Work out the finished part from the listing and answer in its coordinate system (mm). A direction names the side the tool comes from. Coordinates: 2 decimals unless noted, no trailing zeros. Write each loop counter-clockwise with the first axis right and the second up, starting at its lowest first coordinate (ties: lowest second). Pieces come first, ordered by that corner, then holes. Notation, with made-up numbers: (-19, 82.5) - (-7, 82.5) arc R26 ccw to (-7, 98.5) - close; hole circle Ø1 at (-3, 60). An arc over 180 degrees is marked (long way). Use a Markdown table: item, result. Add a question column.
(1) Find the intervals of material crossed by line 1 (Y direction, x = -4, z = -0.75); line 2 (X direction, y = 8, z = -1); line 3 (X direction, y = 23, z = -1.75), in increasing order. Write a range as from..to.
(2) The part is cut by section D-D, the plane x = -16. Give the vertices of the cut face in (y, z).
(3) For a pull along X with two mould halves and no side action, classify faces 1 (the face through (-0.75, 35, 2)), 2 (the face through (0, 17, 0)), 3 (the face through (-21, 3, 0)), 4 (the face through (-5, 37.5, 0)) as released by +X, released by -X, zero draft, split by the parting line, or undercut.
(4) The part is cut by section A-A, the plane y = 33. Give the vertices of the cut face in (x, z), then the cut area to 3 significant figures.
(5) The part is cut by section C-C, the plane x = 2. Give the vertices of the cut face in (y, z).
(6) The part is cut by section B-B, the plane z = 0. Give the vertices of the cut face in (x, y), then the cut area to 3 significant figures.
(7) Given pin 1 Ø4.5 at (y, z) = (34.5, 0.5) entering from -X; pin 2 Ø5.5 at (x, z) = (-18, -2.5) entering from +Y; pin 3 Ø4 at (y, z) = (27.5, 3) entering from +X, each flat-ended and moving along its own axis, determine where each tip first touches the part or whether it passes through.
(8) A tool of negligible diameter and unlimited length cuts with its end or side. For faces 5 (the face through (13, 6, 0)), 6 (the face through (0.75, 35, 2)), 7 (the face through (18.747, 3.042, 0.121)), 8 (the face through (-13, 6, 0)), from which of +Z, -Z, +X, -X, +Y, -Y can it reach the whole face along a straight path? Write none if from no direction.
from build123d import *

# Parameters (mm, degrees)
BOSS_EXTRUDE1_DEPTH = 7
SKETCH2_R           = 6
CUT_EXTRUDE1_DEPTH  = 46.202322949
SKETCH3_R           = 2.05
CUT_EXTRUDE2_DEPTH  = 50.155365933
SKETCH4_R           = 2.75
CUT_EXTRUDE3_DEPTH  = 14
SKETCH5_W           = 1.5
SKETCH5_H           = 29
CUT_EXTRUDE4_DEPTH  = 46.202322949


with BuildPart() as part:
    # Sketch1 → Boss-Extrude1 (new, symmetric)
    with BuildSketch(Plane.XY):
        Polygon((0, 0), (21, 0), (21, 6), (10, 6), (10, 37.5), (0, 37.5), align=None)
    boss_extrude1 = extrude(amount=BOSS_EXTRUDE1_DEPTH, both=True)

    # Mirror1: Boss-Extrude1 across plane
    add(boss_extrude1.mirror(Plane(origin=(0, 37.5, 7), x_dir=(0, 0, 1), z_dir=(1, 0, 0))))

    # Sketch2 → Cut-Extrude1 (cut, through all)
    with BuildSketch(Plane.XY.offset(7)):
        with Locations((0, 23)):
            Circle(SKETCH2_R)
    extrude(amount=-CUT_EXTRUDE1_DEPTH, mode=Mode.SUBTRACT)

    # Sketch3 → Cut-Extrude2 (cut, through all)
    with BuildSketch(Plane(origin=(10, 0, 0), x_dir=(0, 0, -1), z_dir=(1, 0, 0))):
        with Locations((0, 33)):
            Circle(SKETCH3_R)
    extrude(amount=-CUT_EXTRUDE2_DEPTH, mode=Mode.SUBTRACT)

    # Sketch4 → Cut-Extrude3 (cut)
    with BuildSketch(Plane(origin=(0, 6, 0), x_dir=(1, 0, 0), z_dir=(0, 1, 0))):
        with Locations(Location((-16, 0, 0), (0, 0, 180))):
            Circle(SKETCH4_R)
        with Locations(Location((16, 0, 0), (0, 0, 180))):
            Circle(SKETCH4_R)
    extrude(amount=-CUT_EXTRUDE3_DEPTH, mode=Mode.SUBTRACT)

    # Sketch5 → Cut-Extrude4 (cut, through all)
    with BuildSketch(Plane.XY.offset(7)):
        with Locations((0, 37.5)):
            Rectangle(SKETCH5_W, SKETCH5_H)
    extrude(amount=-CUT_EXTRUDE4_DEPTH, mode=Mode.SUBTRACT)


solid = part.part
Model answer:
| question | item | result |
|---|---|---|
| 1 | line 1 | 0..18.53, 27.47..31.09, 34.91..37.5 |
| 1 | line 2 | -10..10 |
| 1 | line 3 | -10..-6, 6..10 |
| 2 | outline | (0, -7) - (6, -7) - (6, -2.75) - (0, -2.75) - close; (0, 2.75) - (6, 2.75) - (6, 7) - (0, 7) - close |
| 3 | face 1 | undercut |
| 3 | face 2 | undercut |
| 3 | face 3 | released by -X |
| 3 | face 4 | zero draft |
| 4 | outline | (-10, -7) - (-0.75, -7) - (-0.75, -2.05) - (-10, -2.05) - close; (-10, 2.05) - (-0.75, 2.05) - (-0.75, 7) - (-10, 7) - close; (0.75, -7) - (10, -7) - (10, -2.05) - (0.75, -2.05) - close; (0.75, 2.05) - (10, 2.05) - (10, 7) - (0.75, 7) - close |
| 4 | area | 183 mm^2 |
| 5 | outline | (0, -7) - (17.34, -7) - (17.34, 7) - (0, 7) - close; (28.66, -7) - (37.5, -7) - (37.5, 7) - (28.66, 7) - close; hole circle Ø4.1 at (33, 0) |
| 6 | outline | (-21, 0) - (-18.75, 0) - (-18.75, 6) - (-21, 6) - close; (-13.25, 0) - (13.25, 0) - (13.25, 6) - (10, 6) - (10, 30.95) - (0.75, 30.95) - (0.75, 28.95) arc R6 cw (long way) to (-0.75, 28.95) - (-0.75, 30.95) - (-10, 30.95) - (-10, 6) - (-13.25, 6) - close; (-10, 35.05) - (-0.75, 35.05) - (-0.75, 37.5) - (-10, 37.5) - close; (0.75, 35.05) - (10, 35.05) - (10, 37.5) - (0.75, 37.5) - close; (18.75, 0) - (21, 0) - (21, 6) - (18.75, 6) - close |
| 6 | area | 614 mm^2 |
| 7 | pin 1 | x = -10 |
| 7 | pin 2 | y = 6 |
| 7 | pin 3 | x = 10 |
| 8 | face 5 | +Z, -Z, +X, +Y |
| 8 | face 6 | +Z, -Z, +Y |
| 8 | face 7 | +Y, -Y |
| 8 | face 8 | +Z, -Z, -X, +Y |
